Part model, mm, in its own coordinate system. Face numbers are marked on the shaded views. A direction names the side the tool comes from. Coordinates: 2 decimals unless noted, no trailing zeros. Order: outer loops, then holes, each group sorted by start corner. A loop starts at its lowest first (then second) coordinate and runs counter-clockwise, first axis right, second up.
1) Mould opens along Y. For the marked faces 5, 6 and 7 say: +Y half, -Y half, draft (parallel to the pull), parting line (faces both ways), or undercut.
2) Tool access for the marked faces 1, 2, 3 and 4: list every direction of +Z, -Z, +X, -X, +Y, -Y with a clear straight run to the whole face (end or side of a thin tool).
3) Wall check: L1, parallel to X at y = -24.5, z = 3.7; L2, parallel to X at y = -22.05, z = -11; L3, parallel to Y at x = 0.5, z = 0.5. Give the ranges that are in metal, low to high.
4) Cut at C-C (z = -11). List the corners of the cut face in (x, y), and give its area (3 significant figures).
5) Pin check, flat tips, straight feed: pin 1 Ø5 at (x, z) = (-4, -12) entering from -Y; pin 2 Ø10 at (x, y) = (-5, 9) entering from +Z; pin 3 Ø6 at (x, z) = (2.5, -5.5) entering from +Y; pin 4 Ø0.7 at (x, y) = (-11.5, -16) entering from -Z. Stop position of each tip, or through.
6) Cut at A-A (y = 1). List the corners of the cut face in (x, z), and give its area (3 significant figures).
7) Cut at D-D (y = 21.5). List the corners of the cut face in (x, z).
8) Cut at B-B (x = 4.15). Give the number of separate pieces and of enclosed holes in the cut face, and give its area (3 significant figures).
Autodesk Inventor part; units mm, degrees
ref_plane "Work Plane2" through (0, -28.5, 5) normal (1, 0, 0) x (0, 0, -1)
ref_plane "YZ Plane" through (0, 0, 0) normal (1, 0, 0) x (0, 1, 0)
ref_plane "XZ Plane" through (0, 0, 0) normal (0, 1, 0) x (-1, 0, 0)
sketch "Sketch1" plane through (0, 0, 0) normal (0, 0, 1) x (1, 0, 0)
  line L0 (-12.5, 28.5) -> (12.5, 28.5)
  line L1 (12.5, 28.5) -> (12.5, -28.5)
  line L2 (12.5, -28.5) -> (-12.5, -28.5)
  line L3 (-12.5, -28.5) -> (-12.5, 28.5)
  line L4 (-10.05, 20.15) -> (10.05, 20.15)
  line L5 (10.05, 20.15) -> (10.05, -20.15)
  line L6 (10.05, -20.15) -> (-10.05, -20.15)
  line L7 (-10.05, -20.15) -> (-10.05, 20.15)
  line L8 (0, 0) -> (0, 17.7516) construction
  line L9 (0, 0) -> (17.0454, 0) construction
  line L10 (-12.5, -28.5) -> (12.5, -28.5)
  line L11 (12.5, -28.5) -> (12.5, -20.15)
  line L12 (12.5, -20.15) -> (-12.5, -20.15)
  line L13 (-12.5, -20.15) -> (-12.5, -28.5)
  circle A0 centre (-4.65, 24.5) radius 2.175
  circle A1 centre (4.65, 24.475) radius 2.175
  circle A2 centre (-4.6492, -24.5) radius 2.175
  circle A3 centre (4.65, -24.375) radius 2.175
  point P0 (12.5, -24.325)
  dimension "d0" = 40.3
  dimension "d1" = 20.1
  dimension "d2" = 57
  dimension "d3" = 25
  dimension "d4" = 4.35
  dimension "d5" = 4.325
  dimension "d6" = 4.35
  dimension "d8" = 4.35
  dimension "d9" = 5.4
  dimension "d13" = 5.4
  dimension "d28" = 48.85
  dimension "d29" = 9.3
  dimension "d30" = 9.3
extrude "Extrusion1" add sketch "Sketch1" along normal blind 5 contours L0 L1 L12 L5 L4 L7 L3 | L12 L6 L1 L2 L3
extrude "Extrusion2" add sketch "Sketch1" against normal blind 15 contours L12 L6 L1 L2 L3 | A2 | A3
extrude "Extrusion3" cut sketch "Sketch1" against normal blind 10 from surface at 5 contours A2 | A3
sketch "Sketch2" plane through (-10.05, -20.15, 5) normal (0, 1, 0) x (1, 0, 0)
  circle A0 centre (5.9, 16) radius 1.1
  circle A1 centre (14.2, 16) radius 1.1
  line L0 (0, 0) -> (20.1, 0) construction
  line L1 (10.05, 0) -> (10.05, 23.167) construction
  line L2 (-2.45, 20) -> (22.55, 20)
  circle A2 centre (14.2, 16) radius 2
  circle A3 centre (5.9, 16) radius 2
  point P0 (10.05, 5)
  dimension "d20" = 2.2
  dimension "d21" = 8.3
  dimension "d22" = 4
  dimension "d23" = 4
extrude "Extrusion4" cut sketch "Sketch2" against normal blind 10 contours A0 | A1
extrude "Extrusion5" cut sketch "Sketch2" against normal blind 3 contours A0 | A1 | A2 | A3
sketch "Sketch3" plane through (12.5, -20.15, 0) normal (1, 0, 0) x (0, 0, -1)
  line L0 (0, 48.65) -> (-5, 48.65) construction
  line L1 (-5, 48.65) -> (38.6712, 48.65) construction
  line L2 (0, 0) -> (-5, 0) construction
  line L3 (-5, 0) -> (38.6712, 0) construction
  line L4 (0, 20) -> (15, 0)
  line L5 (0, 20) -> (0, 13.3333)
  line L6 (0, 13.3333) -> (10, 0)
  line L7 (10, 0) -> (15, 0)
  line L8 (15, 0) -> (15, -8.35) construction
  line L9 (15, -0.9137) -> (15, 2.4866) construction
  line L10 (-5, 0) -> (15, 0)
  line L11 (15, 0) -> (15, -17.35)
  line L12 (15, -17.35) -> (-5, -17.35)
  line L13 (-5, -17.35) -> (-5, 0)
  circle A0 centre (5, -13.35) radius 1.25
  line L14 (0, 0) -> (0, 48.65)
  line L15 (0, 48.65) -> (0, 0)
  line L16 (0, 0) -> (15, 0)
  line L17 (15, -8.35) -> (15, 0)
  line L18 (15, -8.35) -> (-5, -8.35)
  line L19 (-5, 48.65) -> (-5, -8.35)
  line L20 (0, 48.65) -> (-5, 48.65)
  point P0 (0, 20.15)
  dimension "d31" = 4
  dimension "d39" = 2.5
  dimension "d41" = 10
  dimension "d46" = 5
  dimension "d59" = 9
  dimension "d63" = 20
extrude "Extrusion6" add sketch "Sketch3" against normal up to surface (2.45 mm away) contours L4 L7 L6 L5
extrude "Extrusion7" add sketch "Sketch3" along normal blind 4.35 from surface at -25 contours L11 L18 L13 L10 L7 | L11 L12 L13 L18 | A0
extrude "Extrusion8" cut sketch "Sketch3" against normal blind 35.65 contours A0
ref_plane "Work Plane2" through (0, -28.5, 5) normal (1, 0, 0) x (0, 0, -1)
mirror "Mirror1" about plane through (0, -28.5, 5) normal (1, 0, 0) of "Extrusion6"
fillet "Fillet1" radius 1.5 6 edges at (11.275, -20.15, 0) (11.275, -6.8167, 0) (11.275, -20.15, -10) (-11.275, -20.15, -10) (-11.275, -6.8167, 0) (-11.275, -20.15, 0)
chamfer "Chamfer1" distance 1.5 angle 45 3 edges at (12.5, -24.325, -15) (12.5, -10.15, -7.5) (12.5, 14.175, 0)
sketch "Sketch4" plane through (-12.5, 28.5, 0) normal (-1, 0, 0) x (0, 0, 1)
  circle A0 centre (-5, -62) radius 1.25
  circle A1 centre (-5, -62) radius 2
  point P0 (0, -28.5)
  dimension "d51" = 4
extrude "Extrusion9" cut sketch "Sketch4" against normal blind 3
sketch "Sketch5" plane through (-10.05, -20.15, 5) normal (0, 1, 0) x (1, 0, 0)
  line L0 (1.9008, 7.5) -> (8.9008, 7.5)
  line L1 (8.9008, 7.5) -> (8.9008, 4)
  line L2 (8.9008, 4) -> (1.9008, 4)
  line L3 (1.9008, 4) -> (1.9008, 7.5)
  line L4 (11.2, 7.5) -> (18.2, 7.5)
  line L5 (18.2, 7.5) -> (18.2, 4)
  line L6 (18.2, 4) -> (11.2, 4)
  line L7 (11.2, 4) -> (11.2, 7.5)
  line L8 (22.55, 0) -> (-2.45, 0)
  line L9 (5.4008, 4) -> (5.4008, 0) construction
  line L10 (14.7, 4) -> (14.7, 0) construction
  line L11 (7.5758, 0) -> (3.2258, 0) construction
  line L12 (16.875, 0) -> (12.525, 0) construction
  dimension "d54" = 7
  dimension "d55" = 3.5
  dimension "d56" = 4
extrude "Extrusion10" cut sketch "Sketch5" against normal blind 10
chamfer "Chamfer2" distance 9 angle 45 1 edges at (-10.325, -37.5, -15)
equation "\"d8\" = d6"
equation "\"d13\" = d9"
properties part number "BIGServoHolder_3DPrint"
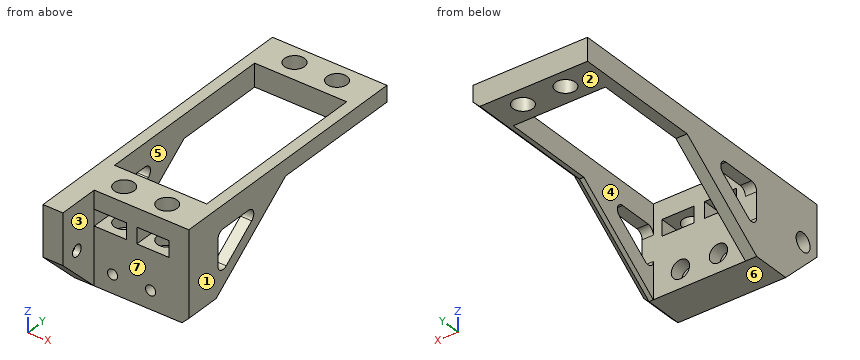
Geometry check:
1. face 5: undercut
1. face 6: draft
1. face 7: -Y half
2. face 1: +Z, -Z, +X, +Y, -Y
2. face 2: -Z, +X, -X, +Y
2. face 3: +Z, -Z, +X, -Y
2. face 4: +Z, -Z
3. L1: x = -12.5 to -6.82, -2.47 to 2.48, 6.82 to 12.5
3. L2: x = -12.5 to -6.15, -2.15 to 2.15, 6.15 to 12.5
3. L3: y = -28.5 to -20.15, 20.15 to 28.5
4. outline: (-12.5, -32.5) - (-8.15, -32.5) - (-8.15, -28.5) - (-5.25, -28.5) - (-5.25, -23.15) - (-6.15, -23.15) - (-6.15, -20.15) - (-10.05, -20.15) - (-10.05, -14.82) - (-12.5, -14.82) - close; (-3.05, -28.5) - (3.05, -28.5) - (3.05, -23.15) - (2.15, -23.15) - (2.15, -20.15) - (-2.15, -20.15) - (-2.15, -23.15) - (-3.05, -23.15) - close; (5.25, -28.5) - (12.5, -28.5) - (12.5, -17.32) - (11, -14.82) - (10.05, -14.82) - (10.05, -20.15) - (6.15, -20.15) - (6.15, -23.15) - (5.25, -23.15) - close
4. area: 203 mm2
5. pin 1: stops at y = -28.5
5. pin 2: passes through
5. pin 3: stops at y = -20.15
5. pin 4: stops at z = -12.15
6. outline: (-12.5, 0) - (-10.05, 0) - (-10.05, 5) - (-12.5, 5) - close; (10.05, 0) - (11, 0) - (12.5, 1.5) - (12.5, 5) - (10.05, 5) - close
6. area: 23.4 mm2
7. outline: (-12.5, 0) - (11, 0) - (12.5, 1.5) - (12.5, 5) - (-12.5, 5) - close
8. separate pieces: 6
8. enclosed holes: 0
8. area: 107 mm2
